Job drawing, mm, ordinate dimensions from the low corner. One solid piece. Give positions to 0.01 mm unless a question says otherwise; leave off trailing zeros. Write each loop counter-clockwise with the first axis right and the second up, starting at its lowest first coordinate (ties: lowest second). Pieces come first, ordered by that corner, then holes. Notation, with made-up numbers: M 70,85 L 110,85 A16 ccw 110,98 Z; hole C -14,-26 d10. An arc over 180 degrees is marked long. Use a Markdown table: item, result.
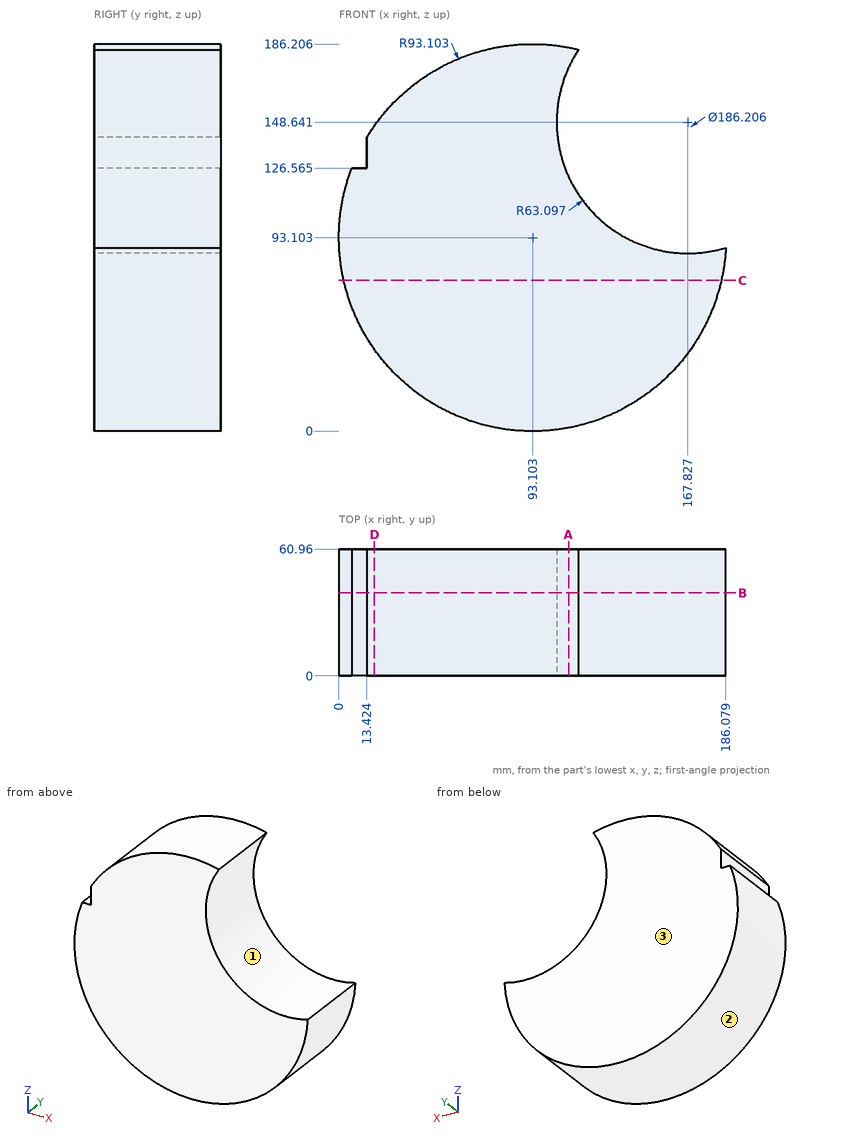
1. Two-plate mould, pull along X, no slides. Class the marked faces 1, 2 and 3: released by +X, released by -X, zero draft, split by the parting line, or undercut.
Findings below:
| item | result |
|---|---|
| face 1 | undercut |
| face 2 | split by the parting line |
| face 3 | zero draft |
2. Cut at D-D, the plane x = 17. Give the cut face in (y, z), then the cut area to 3 significant figures.
Findings below:
| item | result |
|---|---|
| outline | M 0,39.47 L 60.96,39.47 L 60.96,146.74 L 0,146.74 Z |
| area | 6,540 mm2 |
3. Drill centre lines: L1, parallel to Z at x = 117, y = 42 (1 decimal); L2, parallel to Z at x = 99.5, y = 52; L3, parallel to X at y = 10, z = 112.5. Where is each one in solid material? Low to high.
Findings below:
| item | result |
|---|---|
| L1 | 3.1 to 111.3 |
| L2 | 0.22 to 185.99 |
| L3 | 2.04 to 116.11 |
4. Drop flat-ended pins along their axis: P1, Ø5, axis at x = 85, y = 12, coming from the +Z side; P2, Ø8, axis at x = 107, y = 33.5, coming from the +Z side; P3, Ø5, axis at x = 43.5, y = 39, coming from the -Z side (1 decimal). Give the stop position or say it passes through.
Findings below:
| item | result |
|---|---|
| P1 | z = 186.04 |
| P2 | z = 185.68 |
| P3 | z = 12.8 |
5. Cut at A-A, the plane x = 110.5. Give the cut face in (y, z).
Findings below:
| item | result |
|---|---|
| outline | M 0,1.64 L 60.96,1.64 L 60.96,122.28 L 0,122.28 Z; M 0,175 L 60.96,175 L 60.96,184.57 L 0,184.57 Z |
6. Cut at C-C, the plane z = 72.5. Give the cut face in (x, y).
Findings below:
| item | result |
|---|---|
| outline | M 2.31,0 L 183.9,0 L 183.9,60.96 L 2.31,60.96 Z |
7. Cut at B-B, the plane y = 40. Give the cut face in (x, z) (1 decimal).
Findings below:
| item | result |
|---|---|
| outline | M 6.2,126.6 A93.1 ccw long 186.1,88.2 A63.1 cw 115.3,183.5 A93.1 ccw 13.4,141.3 L 13.4,126.6 Z |
